Model file for the job. Use its own axes, mm. Face numbers are marked on the shaded views. A direction names the side the tool comes from. Round coordinates to 2 decimals unless told otherwise and drop trailing zeros. Write each loop counter-clockwise with the first axis right and the second up, starting at its lowest first coordinate (ties: lowest second). Pieces come first, ordered by that corner, then holes. Notation, with made-up numbers: (2.25, -7.75) - (57.25, -7.75) arc R13 ccw to (57.25, 2.25) - close; hole circle Ø7 at (39.25, 66.5). An arc over 180 degrees is marked (long way). One line per item, written item: value.
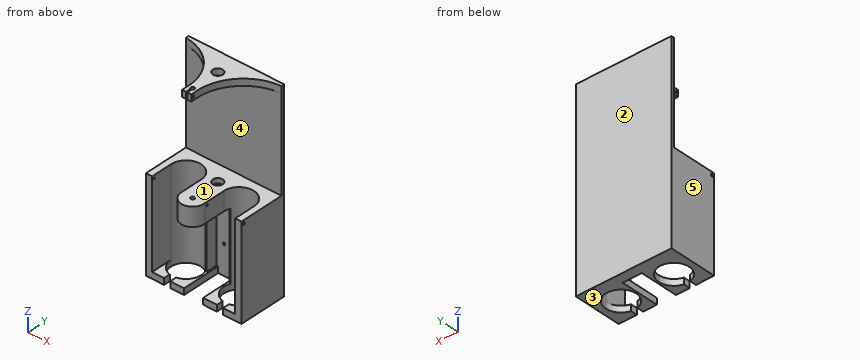
from build123d import *

# Parameters (mm, degrees)
SKETCH1_R                                           = 3
SKETCH1_R_2                                         = 8
BOSS_EXTRUDE1_DEPTH                                 = 30
BOSS_EXTRUDE2_DEPTH                                 = 120
SKETCH5_W                                           = 153.62
SKETCH5_H                                           = 9
SKETCH5_H_2                                         = 6
BOSS_EXTRUDE3_DEPTH                                 = 150
SKETCH6_W                                           = 153.62
SKETCH6_H                                           = 6
BOSS_EXTRUDE4_DEPTH                                 = 150
BOSS_EXTRUDE5_DEPTH                                 = 10.65
CUT_EXTRUDE1_REACH                                  = 337.773
SKETCH8_R                                           = 3
SKETCH8_R_2                                         = 8
SKETCH9_R                                           = 13.5
CUT_EXTRUDE2_DEPTH                                  = 22
SKETCH10_R                                          = 2
CUT_EXTRUDE3_DEPTH                                  = 6.7
SKETCH12_W                                          = 40.684038992
SKETCH12_H                                          = 10
CUT_EXTRUDE5_DEPTH                                  = 120
BOSS_EXTRUDE6_START                                 = -10
BOSS_EXTRUDE6_DEPTH                                 = 10
SKETCH11_W                                          = 153.62
SKETCH11_H                                          = 10
CUT_EXTRUDE4_DEPTH                                  = 336.773166974
CUT_EXTRUDE6_REACH                                  = 201.52
CUT_EXTRUDE6_END_RADIUS                             = 3
SKETCH14_W                                          = 2
SKETCH14_H                                          = 10.65
CSK_FOR_M2_COUNTERSUNK_FLAT_HEAD_SCREW1_D           = 2.4
CSK_FOR_M2_COUNTERSUNK_FLAT_HEAD_SCREW1_DEPTH       = 16.5
CSK_FOR_M2_COUNTERSUNK_FLAT_HEAD_SCREW1_CSINK_D     = 4.4
CSK_FOR_M2_COUNTERSUNK_FLAT_HEAD_SCREW1_CSINK_ANGLE = 90
CSK_FOR_M2_COUNTERSUNK_FLAT_HEAD_SCREW1_TIP         = 0.721032743
CUT_EXTRUDE7_DEPTH                                  = 1.6
SKETCH22_R                                          = 1.6
CUT_EXTRUDE8_DEPTH                                  = 4
CUT_EXTRUDE9_DEPTH                                  = 1.6
CUT_EXTRUDE10_REACH                                 = 240.276
SKETCH24_R                                          = 1.2


with BuildPart() as part:
    # Sketch1 → Boss-Extrude1 (new body)
    with BuildSketch(Plane.XY):
        with BuildLine():
            Line((-18.19, -47.31), (-18.19, -81.62))
            ThreePointArc((-18.19, -81.62), (0, -101.687860925), (18.19, -81.62))
            Line((18.19, -81.62), (18.19, -47.31))
            ThreePointArc((18.19, -47.31), (42.5, -23), (66.81, -47.31))
            Line((66.81, -47.31), (66.81, -81.62))
            Line((66.81, -81.62), (76.81, -81.62))
            Line((76.81, -81.62), (76.81, 0))
            Line((76.81, 0), (-76.81, 0))
            Line((-76.81, 0), (-76.81, -81.62))
            Line((-76.81, -81.62), (-66.81, -81.62))
            Line((-66.81, -81.62), (-66.81, -47.31))
            ThreePointArc((-66.81, -47.31), (-42.5, -23), (-18.19, -47.31))
        make_face()
        with Locations((0, -83.41)):
            Circle(SKETCH1_R, mode=Mode.SUBTRACT)
        with Locations((0, -37.71)):
            Circle(SKETCH1_R_2, mode=Mode.SUBTRACT)
    extrude(amount=-BOSS_EXTRUDE1_DEPTH)

    # Sketch3 → Boss-Extrude2 (add)
    with BuildSketch(Plane(origin=(0, 0, -30), x_dir=(-1, 0, 0), z_dir=(0, 0, -1))):
        with BuildLine():
            Line((-76.81, 0), (-76.81, -81.62))
            Line((-76.81, -81.62), (-66.81, -81.62))
            Line((-66.81, -81.62), (-66.81, -47.31))
            ThreePointArc((-66.81, -47.31), (-42.5, -23), (-18.19, -47.31))
            Line((-18.19, -47.31), (-18.19, -19.7))
            Line((-18.19, -19.7), (18.19, -19.7))
            Line((18.19, -19.7), (18.19, -47.31))
            ThreePointArc((18.19, -47.31), (42.5, -23), (66.81, -47.31))
            Line((66.81, -47.31), (66.81, -81.62))
            Line((66.81, -81.62), (76.81, -81.62))
            Line((76.81, -81.62), (76.81, 0))
            Line((76.81, 0), (-76.81, 0))
        make_face()
    extrude(amount=BOSS_EXTRUDE2_DEPTH)

    # Sketch5 → Boss-Extrude3 (add)
    with BuildSketch(Plane.XY):
        with Locations((0, -4.5)):
            Rectangle(SKETCH5_W, SKETCH5_H)
        with Locations((0, 3)):
            Rectangle(SKETCH5_W, SKETCH5_H_2)
    extrude(amount=BOSS_EXTRUDE3_DEPTH)

    # Sketch6 → Boss-Extrude4 (add)
    with BuildSketch(Plane(origin=(0, 0, 0), x_dir=(-1, 0, 0), z_dir=(0, 0, -1))):
        with Locations((0, 3)):
            Rectangle(SKETCH6_W, SKETCH6_H)
    extrude(amount=BOSS_EXTRUDE4_DEPTH)

    # Sketch7 → Boss-Extrude5 (add)
    with BuildSketch(Plane.XY.offset(150)):
        with BuildLine():
            Line((-76.81, -9), (-76.81, 6))
            Line((-76.81, 6), (76.81, 6))
            Line((76.81, 6), (76.81, -9))
            ThreePointArc((76.81, -9), (25.316346961, -34.411411974), (7.5, -89))
            Line((7.5, -89), (7.5, -94))
            Line((7.5, -94), (-7.5, -94))
            Line((-7.5, -94), (-7.5, -89))
            ThreePointArc((-7.5, -89), (-25.316346961, -34.411411974), (-76.81, -9))
        make_face()
    extrude(amount=BOSS_EXTRUDE5_DEPTH)

    # Sketch8 → Cut-Extrude1 (cut, up to next)
    with BuildSketch(Plane.XY.offset(160.65), mode=Mode.PRIVATE) as cut_extrude1_sk1:
        with Locations((0, -83.41)):
            Circle(SKETCH8_R)
    cut_extrude1_tool1 = extrude(cut_extrude1_sk1.sketch, amount=-CUT_EXTRUDE1_REACH, mode=Mode.PRIVATE) & part.part
    # Sketch8 → Cut-Extrude1 (cut, up to next)
    with BuildSketch(Plane.XY.offset(160.65), mode=Mode.PRIVATE) as cut_extrude1_sk2:
        with Locations((0, -37.71)):
            Circle(SKETCH8_R_2)
    cut_extrude1_tool2 = extrude(cut_extrude1_sk2.sketch, amount=-CUT_EXTRUDE1_REACH, mode=Mode.PRIVATE) & part.part
    add(cut_extrude1_tool1.solids().sort_by_distance((0, -83.41, 160.65))[0], mode=Mode.SUBTRACT)
    add(cut_extrude1_tool2.solids().sort_by_distance((0, -37.71, 160.65))[0], mode=Mode.SUBTRACT)

    # Sketch9 → Cut-Extrude2 (cut)
    with BuildSketch(Plane(origin=(0, 0, -30), x_dir=(-1, 0, 0), z_dir=(0, 0, -1))):
        with Locations((0, -37.71)):
            Circle(SKETCH9_R)
    extrude(amount=-CUT_EXTRUDE2_DEPTH, mode=Mode.SUBTRACT)

    # Sketch10 → Cut-Extrude3 (cut)
    with BuildSketch(Plane.XZ.offset(19.7)):
        with Locations((-6, -102.85)):
            Circle(SKETCH10_R)
        with Locations((6, -102.85)):
            Circle(SKETCH10_R)
    extrude(amount=-CUT_EXTRUDE3_DEPTH, mode=Mode.SUBTRACT)

    # Sketch12 → Cut-Extrude5 (cut)
    with BuildSketch(Plane(origin=(0, 0, -150), x_dir=(-1, 0, 0), z_dir=(0, 0, -1))):
        with Locations((0, -42.31)):
            Rectangle(SKETCH12_W, SKETCH12_H)
    extrude(amount=-CUT_EXTRUDE5_DEPTH, mode=Mode.SUBTRACT)

    # Sketch13 → Boss-Extrude6 (add)
    with BuildSketch(Plane(origin=(0, 0, -150), x_dir=(-1, 0, 0), z_dir=(0, 0, -1)).offset(BOSS_EXTRUDE6_START)):
        with BuildLine():
            Line((-18.19, -37.31), (-20.342019496, -37.31))
            ThreePointArc((-20.342019496, -37.31), (-18.734093684, -42.195530626), (-18.19, -47.31))
            ThreePointArc((-18.19, -47.31), (-23.625068212, -62.630347581), (-37.5, -71.100252205))
            Line((-37.5, -71.100252205), (-37.5, -81.62))
            Line((-37.5, -81.62), (-15.342019496, -81.62))
            Line((-15.342019496, -81.62), (-15.342019496, -37.31))
            Line((-15.342019496, -37.31), (-15.342019496, -19.7))
            Line((-15.342019496, -19.7), (-18.19, -19.7))
            Line((-18.19, -19.7), (-18.19, -37.31))
        make_face()
        with BuildLine():
            ThreePointArc((-47.5, -71.100252205), (-61.374931788, -62.630347581), (-66.81, -47.31))
            Line((-66.81, -47.31), (-66.81, -81.62))
            Line((-66.81, -81.62), (-47.5, -81.62))
            Line((-47.5, -81.62), (-47.5, -71.100252205))
        make_face()
    boss_extrude6 = extrude(amount=BOSS_EXTRUDE6_DEPTH)

    # Sketch11 → Cut-Extrude4 (cut, through all)
    with BuildSketch(Plane.XY.offset(160.65)):
        with Locations((0, 1)):
            Rectangle(SKETCH11_W, SKETCH11_H)
    extrude(amount=-CUT_EXTRUDE4_DEPTH, mode=Mode.SUBTRACT)

    # Mirror1: Boss-Extrude6 across plane
    add(boss_extrude6.mirror(Plane(origin=(0, 0, 0), x_dir=(0, 0, 1), z_dir=(1, 0, 0))))

    # Cut-Extrude6: up to this cylinder (the profile starts outside it)
    cut_extrude6_end = Plane(origin=(0, -83.41, 155.325), z_dir=(0, 0, 1)) * Cylinder(CUT_EXTRUDE6_END_RADIUS, 410.04, mode=Mode.PRIVATE)
    # Sketch14 → Cut-Extrude6 (cut, up to the surface)
    with BuildSketch(Plane.XZ.offset(94), mode=Mode.PRIVATE) as cut_extrude6_sk1:
        with Locations((0, 155.325)):
            Rectangle(SKETCH14_W, SKETCH14_H)
    cut_extrude6_tool1 = extrude(cut_extrude6_sk1.sketch, amount=-CUT_EXTRUDE6_REACH, mode=Mode.PRIVATE) - cut_extrude6_end
    add(cut_extrude6_tool1.solids().sort_by_distance((0, -94, 155.325))[0], mode=Mode.SUBTRACT)

    # CSK for M2 Countersunk Flat Head Screw1
    with Locations(Plane.ZY.offset(7.5)):
        with Locations((155.325, -91.5)):
            CounterSinkHole(CSK_FOR_M2_COUNTERSUNK_FLAT_HEAD_SCREW1_D / 2, CSK_FOR_M2_COUNTERSUNK_FLAT_HEAD_SCREW1_CSINK_D / 2, depth=CSK_FOR_M2_COUNTERSUNK_FLAT_HEAD_SCREW1_DEPTH, counter_sink_angle=CSK_FOR_M2_COUNTERSUNK_FLAT_HEAD_SCREW1_CSINK_ANGLE)
            with Locations((0, 0, -(CSK_FOR_M2_COUNTERSUNK_FLAT_HEAD_SCREW1_DEPTH + CSK_FOR_M2_COUNTERSUNK_FLAT_HEAD_SCREW1_TIP / 2))):  # 118° drill point
                Cone(0, CSK_FOR_M2_COUNTERSUNK_FLAT_HEAD_SCREW1_D / 2, CSK_FOR_M2_COUNTERSUNK_FLAT_HEAD_SCREW1_TIP, mode=Mode.SUBTRACT)

    # Sketch19 → Cut-Extrude7 (cut)
    with BuildSketch(Plane(origin=(7.5, 0, 0), x_dir=(0, 0, -1), z_dir=(1, 0, 0))):
        Polygon((-154.170299462, -93.5), (-153.015598923, -91.5), (-154.170299462, -89.5), (-156.479700538, -89.5), (-157.634401077, -91.5), (-156.479700538, -93.5), align=None)
    extrude(amount=-CUT_EXTRUDE7_DEPTH, mode=Mode.SUBTRACT)

    # Sketch22 → Cut-Extrude8 (cut)
    with BuildSketch(Plane.ZY.offset(18.19)):
        with Locations(Location((-5, -77.65, 0), (0, 0, 270))):
            Circle(SKETCH22_R)
    cut_extrude8 = extrude(amount=-CUT_EXTRUDE8_DEPTH, mode=Mode.SUBTRACT)

    # Mirror2: Cut-Extrude8 across plane
    add(cut_extrude8.mirror(Plane(origin=(0, 0, 0), x_dir=(0, 0, 1), z_dir=(1, 0, 0))), mode=Mode.SUBTRACT)

    # Sketch23 → Cut-Extrude9 (cut)
    with BuildSketch(Plane.ZY.offset(76.81)):
        Polygon((-5, -75.340598923), (-7, -76.495299462), (-7, -78.804700538), (-5, -79.959401077), (-3, -78.804700538), (-3, -76.495299462), align=None)
    cut_extrude9 = extrude(amount=-CUT_EXTRUDE9_DEPTH, mode=Mode.SUBTRACT)

    # Mirror3: Cut-Extrude9 across plane
    add(cut_extrude9.mirror(Plane(origin=(0, 0, 0), x_dir=(0, 0, 1), z_dir=(1, 0, 0))), mode=Mode.SUBTRACT)

    # Sketch24 → Cut-Extrude10 (cut, up to next)
    with BuildSketch(Plane(origin=(-66.81, 0, 0), x_dir=(0, 0, -1), z_dir=(1, 0, 0)), mode=Mode.PRIVATE) as cut_extrude10_sk1:
        with Locations((5, -77.65)):
            Circle(SKETCH24_R)
    cut_extrude10_tool1 = extrude(cut_extrude10_sk1.sketch, amount=-CUT_EXTRUDE10_REACH, mode=Mode.PRIVATE) & part.part
    cut_extrude10 = cut_extrude10_tool1.solids().sort_by_distance((-66.81, -77.65, -5))[0]
    add(cut_extrude10, mode=Mode.SUBTRACT)

    # Mirror4: Cut-Extrude10 across plane
    add(cut_extrude10.mirror(Plane(origin=(0, 0, 0), x_dir=(0, 0, 1), z_dir=(1, 0, 0))), mode=Mode.SUBTRACT)


solid = part.part
1. Tool access for the marked faces 1 and 2: list every direction of +Z, -Z, +X, -X, +Y, -Y with a clear straight run to the whole face (end or side of a thin tool).
Report:
face 1: +X, -X, -Y
face 2: +Z, -Z, +X, -X, +Y
2. Mould opens along Z. For the marked faces 3, 4 and 5 say: released by +Z, released by -Z, zero draft, split by the parting line, or undercut.
Report:
face 3: released by -Z
face 4: undercut
face 5: zero draft
3. Band-saw the part on A-A on x = -30. Write the cut outline in (y, z).
Report:
outline: (-81.62, -150) - (-68.16, -150) - (-68.16, -140) - (-81.62, -140) - close; (-29.48, 150) - (-9, 150) - (-9, 0) - (-26.46, 0) - (-26.46, -150) - (-4, -150) - (-4, 160.65) - (-29.48, 160.65) - close
4. Drop flat-ended pins along their axis: pin 1 (4 mm diameter, centred on y = -91.5, z = 156, fed in from -X); pin 2 (2 mm diameter, centred on y = -78, z = -5, fed in from +X); pin 3 (4.5 mm diameter, centred on x = -6, z = -103, fed in from -Y). Give the stop position or say it passes through.
Report:
pin 1: x = -7.5
pin 2: x = 75.21
pin 3: y = -19.7
5. Band-saw the part on D-D on x = 61.5. Write the cut outline in (y, z), plus the area to 3 significant figures.
Report:
outline: (-81.62, -150) - (-62.47, -150) - (-62.47, -140) - (-81.62, -140) - close; (-32.15, -150) - (-4, -150) - (-4, 160.65) - (-11.55, 160.65) - (-11.55, 150) - (-9, 150) - (-9, 0) - (-32.15, 0) - close
area: 5,240 mm²
6. Band-saw the part on C-C on z = -22. Write the cut outline in (x, y), plus the area to 3 significant figures.
Report:
outline: (-76.81, -81.62) - (-66.81, -81.62) - (-66.81, -47.31) arc R24.31 cw to (-18.19, -47.31) - (-18.19, -81.62) arc R18.28 ccw (long way) to (18.19, -81.62) - (18.19, -47.31) arc R24.31 cw to (66.81, -47.31) - (66.81, -81.62) - (76.81, -81.62) - (76.81, -4) - (-76.81, -4) - close; hole circle Ø27 at (0, -37.71); hole circle Ø6 at (0, -83.41)
area: 6,720 mm²
7. Wall check: probe 1 along X at (y, z) = (-52, -4); probe 2 along Y at (x, z) = (69.5, -5); probe 3 along Y at (x, z) = (0, 153). Give the ranges that are in metal, low to high. Write a range as [from, to].
Report:
probe 1: [-76.81, -66.81], [-18.19, 18.19], [66.81, 76.81]
probe 2: [-81.62, -78.85], [-76.45, -4]
probe 3: [-80.41, -45.71], [-29.71, -4]
8. Band-saw the part on B-B on y = -68. Write the cut outline in (x, z).
Report:
outline: (-76.81, -150) - (-55.26, -150) - (-55.26, -140) - (-66.81, -140) - (-66.81, 0) - (-76.81, 0) - close; (-29.74, -150) - (-15.34, -150) - (-15.34, -140) - (-29.74, -140) - close; (-18.19, -30) - (18.19, -30) - (18.19, 0) - (-18.19, 0) - close; (-8.75, 150) - (8.75, 150) - (8.75, 160.65) - (-8.75, 160.65) - close; (15.34, -150) - (29.74, -150) - (29.74, -140) - (15.34, -140) - close; (55.26, -150) - (76.81, -150) - (76.81, 0) - (66.81, 0) - (66.81, -140) - (55.26, -140) - close
